Part model, mm, in its own coordinate system. A direction names the side the tool comes from. Coordinates: 2 decimals unless noted, no trailing zeros. Order: outer loops, then holes, each group sorted by start corner. A loop starts at its lowest first (then second) coordinate and runs counter-clockwise, first axis right, second up.
Autodesk Inventor part; units mm, degrees
ref_plane "Work Plane1" through (9, 0, 0) normal (1, 0, 0) x (0, 0, -1)
ref_plane "YZ Plane" through (0, 0, 0) normal (1, 0, 0) x (0, 1, 0)
ref_plane "XZ Plane" through (0, 0, 0) normal (0, 1, 0) x (-1, 0, 0)
sketch "Sketch1" plane through (0, 0, 0) normal (1, 0, 0) x (0, 1, 0)
  circle A0 centre (0, 0) radius 1.4
  line L0 (0.5, 1.30767) -> (0.5, -1.30767)
  dimension "d1" = 2.8
  dimension "d2" = 0.5
extrude "Extrusion1" add sketch "Sketch1" along normal blind 8 contours L0 A0 picked at (-0.62029, 0.295862)
sketch "Sketch2" plane through (0, 0, 0) normal (-1, 0, 0) x (0, 0, 1)
  circle A0 centre (0, 0) radius 8.75
  arc A1 (-1.30767, 0.5) -> (1.30767, 0.5) centre (0, 0) ccw
  dimension "d5" = 17.5
extrude "Extrusion2" add sketch "Sketch2" along normal blind 8
sketch "Sketch3" plane through (0, 0, 0) normal (1, 0, 0) x (0, 1, 0)
  circle A0 centre (0, 0) radius 4.25
  line L0 (4, 1.7) -> (8.583269, 1.7)
  line L1 (4, -1.7) -> (8.583269, -1.7)
  line L2 (-10.5, 0) -> (10.5, 0)
  circle A1 centre (0, 0) radius 8.75
  line L3 (0.5, -1.30767) -> (0.5, 1.30767)
  arc A2 (0.5, 1.30767) -> (0.5, -1.30767) centre (0, 0) ccw
  arc A3 (3.852905, 1.793773) -> (4, 1.7) centre (4, 1.862255) ccw
  arc A4 (4, -1.7) -> (3.852905, -1.793773) centre (4, -1.862255) ccw
  line L4 (-3.472243, 2.614102) -> (-5.763877, 6.583329)
  line L5 (-0.527757, 4.314102) -> (-2.819391, 8.283329)
  arc A5 (-0.527757, 4.314102) -> (-0.373, 4.2336) centre (-0.38724, 4.395229) ccw
  arc A6 (-3.479906, 2.439827) -> (-3.472243, 2.614102) centre (-3.61276, 2.532974) ccw
  line L6 (-0.527757, -4.314102) -> (-2.819391, -8.283329)
  line L7 (-3.472243, -2.614102) -> (-5.763877, -6.583329)
  arc A7 (-3.472243, -2.614102) -> (-3.479906, -2.439827) centre (-3.61276, -2.532974) ccw
  arc A8 (-0.373, -4.2336) -> (-0.527757, -4.314102) centre (-0.38724, -4.395229) ccw
  arc A9 (0.5, 1.30767) -> (0.5, -1.30767) centre (0, 0) ccw
  circle A10 centre (0, 0) radius 5
  line L8 (4, 1.7) -> (3.895189, 1.7)
  line L9 (4, -1.7) -> (3.840573, -1.7)
  line L10 (-0.527757, -4.314102) -> (-0.475351, -4.223333)
  line L11 (-3.472243, -2.614102) -> (-3.419838, -2.523333)
  line L12 (-3.472243, 2.614102) -> (-3.419838, 2.523333)
  line L13 (-0.527757, 4.314102) -> (-0.475351, 4.223333)
  point P0 (-3.479906, -2.439827)
  point P1 (-4.25, 0)
  point P2 (-8.75, 0)
  point P3 (-0.373, -4.2336)
  point P4 (-2.819391, -8.283329)
  point P5 (-0.373, 4.2336)
  point P6 (-2.819391, 8.283329)
  point P7 (-3.479906, 2.439827)
  point P8 (3.895189, -1.7)
  dimension "d8" = 8.5
  dimension "d9" = 3.4
  dimension "d10" = 4
  dimension "d14" = 360
  dimension "d22" = 10
extrude "Extrusion3" add sketch "Sketch3" along normal blind 8 contours A0 A3 L8 | L9 A4 A0 | A0 A5 L5 A10 L0 A3 | A4 L1 A10 L6 A8 A0 | A10 L5 A1 L0 | L1 A1 L6 A10 | A0 L13 A5 | A8 L10 A0 | L2 A10 L4 A6 A0 | A0 A7 L7 A10 L2 | A10 L2 A1 L4 | L7 A1 L2 A10 | A6 L12 A0 | A0 L11 A7
sketch "Sketch4" plane through (-8, 0, 0) normal (-1, 0, 0) x (0, 0, 1)
  circle A0 centre (0, 0) radius 6.65
  dimension "d19" = 13.3
extrude "Extrusion4" cut sketch "Sketch4" against normal blind 7
fillet "Fillet1" radius 3 6 edges at (4, 3.8952, 1.7) (4, -0.4754, 4.2233) (4, 3.8952, -1.7) (4, -0.4754, -4.2233) (4, -3.4198, -2.5233) (4, -3.4198, 2.5233)
sketch "Sketch5" plane through (-1, 0, 0) normal (-1, 0, 0) x (0, 0, 1)
  circle A0 centre (0, 0) radius 2.5
  dimension "d24" = 5
extrude "Extrusion5" [suppressed]
sketch "Sketch6" plane through (-22, 0, 0) normal (-1, 0, 0) x (0, 0, 1)
  arc A0 (-1.2, 0.5) -> (1.2, 0.5) centre (0, 0) ccw
  circle A1 centre (0, 0) radius 2.5
ref_plane "Work Plane1" through (9, 0, 0) normal (1, 0, 0) x (0, 0, -1)
sketch "Sketch7" plane through (9, 0, 0) normal (1, 0, 0) x (0, 0, -1)
  arc A0 (-1.30767, 0.5) -> (1.30767, 0.5) centre (0, 0) ccw
  line L0 (1.30767, 0.5) -> (-1.30767, 0.5)
  circle A1 centre (0, 0) radius 1.6
  line L1 (-1.438749, 0.7) -> (1.438749, 0.7)
  dimension "d28" = 3.2
  dimension "d30" = 0.5
  dimension "d31" = 0.7
sketch "Sketch8" plane through (8, 0, 0) normal (1, 0, 0) x (0, 0, -1)
  arc A0 (-1.30767, 0.5) -> (1.30767, 0.5) centre (0, 0) ccw
  line L0 (1.30767, 0.5) -> (-1.30767, 0.5)
sketch "Sketch7 outline for Loft1" plane through (9, 0, 0) normal (1, 0, 0) x (0, 0, -1)
  line L0 (1.438749, 0.7) -> (-1.438749, 0.7)
  arc A0 (-1.438749, 0.7) -> (1.438749, 0.7) centre (0, 0) ccw
loft "Loft1" add profiles "Sketch7 outline for Loft1" section 1 edges at (8, -1.4, 0) (8, 0.5, 0)
properties part number "front wheel mount"
Q1. Which spindle directions (+Z, -Z, +X, -X, +Y, -Y) get a long thin tool onto all of the face, cutting with end or side? Do faces 1 (the face through (8, 3, -5)), 2 (the face through (4, 7, -1.7)), 3 (the face through (3.944, -2.043, 6.938)). Say none if no direction does.
Results list:
face 1: -Z, +X, +Y, -Y
face 2: +X, +Y
face 3: +X
Q2. Wall check: line 1 along Y through (x, z) = (-4, 0); line 2 along X through (y, z) = (5.25, 2); line 3 along Y through (x, z) = (4.5, 1). Give the ranges that are in metal, low to high.
Results list:
line 1: y = -8.75 to -6.65, 6.65 to 8.75
line 2: x = -1 to 8
line 3: y = -8.69 to -4.13, -0.98 to 0.5
Q3. Mould opens along X. For faces 4 (the face through (8, 3, 5)), 5 (the face through (3.9, -1.4, 0)), 6 (the face through (3.944, -2.043, -6.938)) say: pulls with the +X half, pulls with the -X half, needs draft (parallel to the pull), parting line crosses it, or undercut.
Results list:
face 4: pulls with the +X half
face 5: undercut
face 6: needs draft
Q4. Cut at A-A on x = 2.5. Write the cut outline in (y, z), and give its area (3 significant figures).
Results list:
outline: (-5.76, -6.58) - (-4.23, -3.93) arc R3 ccw to (-4, -1.42) arc R4.25 cw to (-4, 1.42) arc R3 ccw to (-4.23, 3.93) - (-5.76, 6.58) arc R8.75 ccw to start; (-2.82, -8.28) arc R8.75 ccw to (8.58, -1.7) - (5.52, -1.7) arc R3 ccw to (3.24, -2.76) arc R4.25 cw to (0.77, -4.18) arc R3 ccw to (-1.29, -5.63) - close; (-2.82, 8.28) - (-1.29, 5.63) arc R3 ccw to (0.77, 4.18) arc R4.25 cw to (3.24, 2.76) arc R3 ccw to (5.52, 1.7) - (8.58, 1.7) arc R8.75 ccw to start; (0.5, -1.31) - (0.5, 1.31) arc R1.4 ccw (long way) to start
area: 140 mm2
Q5. Pin check, flat tips, straight feed: pin 1 Ø0.8 at (x, z) = (5, 0) entering from +Y; pin 2 Ø2.5 at (y, z) = (-6.5, -3.5) entering from +X; pin 3 Ø1 at (x, y) = (-3, -5) entering from -Z. Stop position of each tip, or through.
Results list:
pin 1: stops at y = 0.5
pin 2: stops at x = 8
pin 3: stops at z = -7.5
Q6. Cut at B-B on y = -3.25. Write the cut outline in (x, z), and give its area (3 significant figures).
Results list:
outline: (-8, -8.12) - (0, -8.12) - (0, 8.12) - (-8, 8.12) - (-8, 5.8) - (-1, 5.8) - (-1, -5.8) - (-8, -5.8) - close
area: 48.8 mm2
